Part model, mm, in its own coordinate system. Face numbers are marked on the shaded views. A direction names the side the tool comes from. Coordinates: 2 decimals unless noted, no trailing zeros. Write each loop counter-clockwise with the first axis right and the second up, starting at its lowest first coordinate (ties: lowest second). Pieces come first, ordered by that corner, then holes. Notation, with made-up numbers: (-23, 69) - (25, 69) arc R20 ccw to (25, 98) - close; hole circle Ø6 at (67.25, -17.75). An arc over 180 degrees is marked (long way). Use a Markdown table: item, result.
```python
from build123d import *

# Parameters (mm, degrees)
SKETCH1_R           = 15
SKETCH1_R_2         = 10
BOSS_EXTRUDE1_DEPTH = 5
BOSS_EXTRUDE2_DEPTH = 9.5
FILLET1_R           = 0.5


with BuildPart() as part:
    # Sketch1 → Boss-Extrude1 (new body)
    with BuildSketch(Plane.XY):
        Circle(SKETCH1_R)
        Circle(SKETCH1_R_2, mode=Mode.SUBTRACT)
    extrude(amount=BOSS_EXTRUDE1_DEPTH)

    # Sketch1_3 → Boss-Extrude2 (add)
    with BuildSketch(Plane.XY):
        with BuildLine():
            Line((-9.797958971, 2), (-2, 2))
            Line((-2, 2), (-2, 9.797958971))
            ThreePointArc((-2, 9.797958971), (-7.071067812, 7.071067812), (-9.797958971, 2))
        make_face()
        with BuildLine():
            Line((2, 9.797958971), (2, 2))
            Line((2, 2), (9.797958971, 2))
            ThreePointArc((9.797958971, 2), (7.071067812, 7.071067812), (2, 9.797958971))
        make_face()
        with BuildLine():
            Line((2, -2), (2, -9.797958971))
            ThreePointArc((2, -9.797958971), (7.071067812, -7.071067812), (9.797958971, -2))
            Line((9.797958971, -2), (2, -2))
        make_face()
        with BuildLine():
            ThreePointArc((-9.797958971, -2), (-7.071067812, -7.071067812), (-2, -9.797958971))
            Line((-2, -9.797958971), (-2, -2))
            Line((-2, -2), (-9.797958971, -2))
        make_face()
    extrude(amount=BOSS_EXTRUDE2_DEPTH)

    # Fillet1
    fillet1_edges = [part.edges().sort_by_distance(p)[0] for p in [
        (-2, 5.898979486, 0),
        (-5.898979486, 2, 0),
        (0, 10, 0),
        (5.898979486, 2, 0),
        (2, 5.898979486, 0),
        (10, 0, 0),
        (2, -5.898979486, 0),
        (5.898979486, -2, 0),
        (0, -10, 0),
        (-2, -5.898979486, 0),
        (-5.898979486, -2, 0),
        (-10, 0, 0),
    ]]
    fillet(fillet1_edges, radius=FILLET1_R)


solid = part.part
```
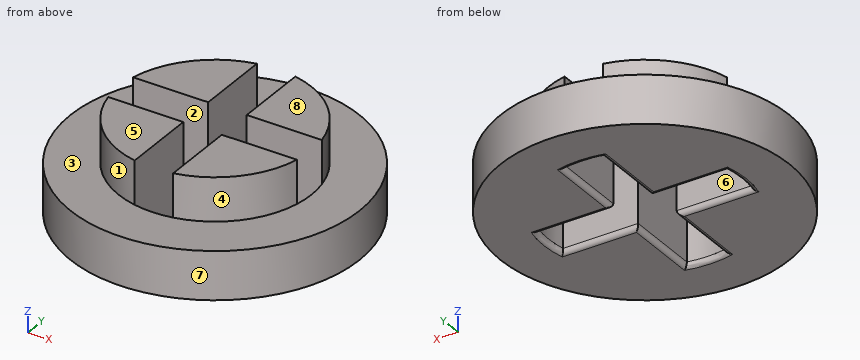
Item 1: Band-saw the part on A-A, the plane z = 3.25. Give the cut face in (x, y).
From the geometry:
| item | result |
|---|---|
| outline | circle Ø30 at (0, 0); hole (-9.8, -2) - (-2, -2) - (-2, -9.8) arc R10 ccw to (2, -9.8) - (2, -2) - (9.8, -2) arc R10 ccw to (9.8, 2) - (2, 2) - (2, 9.8) arc R10 ccw to (-2, 9.8) - (-2, 2) - (-9.8, 2) arc R10 ccw to start |
Item 2: Two-plate mould, pull along X, no slides. Class the marked faces 6, 7 and 8: pulls with the +X half, pulls with the -X half, needs draft (parallel to the pull), parting line crosses it, or undercut.
From the geometry:
| item | result |
|---|---|
| face 6 | undercut |
| face 7 | parting line crosses it |
| face 8 | needs draft |
Item 3: Drop flat-ended pins along their axis: P1, Ø2.5, axis at y = -6.5, z = 5.5, coming from the +X side; P2, Ø1.5, axis at y = 3.5, z = 3.5, coming from the -X side; P3, Ø3, axis at x = -2, z = 6, coming from the -Y side. Give the stop position or say it passes through.
From the geometry:
| item | result |
|---|---|
| P1 | x = 14.01 |
| P2 | x = -14.75 |
| P3 | y = -14.97 |
Item 4: Drill centre lines: probe 1 along Y at (x, z) = (0, 1); probe 2 along Y at (x, z) = (3.5, 7.75); probe 3 along Z at (x, y) = (13, -0.25). Where is each one in solid material? Low to high.
From the geometry:
| item | result |
|---|---|
| probe 1 | -15 to -10, 10 to 15 |
| probe 2 | -9.37 to -2, 2 to 9.37 |
| probe 3 | 0 to 5 |
Item 5: Band-saw the part on C-C, the plane z = 8. Give the cut face in (x, y).
From the geometry:
| item | result |
|---|---|
| outline | (-9.8, -2) arc R10 ccw to (-2, -9.8) - (-2, -2) - close; (-9.8, 2) - (-2, 2) - (-2, 9.8) arc R10 ccw to start; (2, -9.8) arc R10 ccw to (9.8, -2) - (2, -2) - close; (2, 2) - (9.8, 2) arc R10 ccw to (2, 9.8) - close |
Item 6: Which spindle directions (+Z, -Z, +X, -X, +Y, -Y) get a long thin tool onto all of the face, cutting with end or side? Do the marked faces 1, 2, 3, 4 and 5. Say none if no direction does.
From the geometry:
| item | result |
|---|---|
| face 1 | +Z, -X, -Y |
| face 2 | +Z, -Z |
| face 3 | +Z |
| face 4 | +Z, +X, -Y |
| face 5 | +Z, +X, -X, +Y, -Y |
Item 7: Band-saw the part on B-B, the plane y = 0. Give the cut face in (x, z).
From the geometry:
| item | result |
|---|---|
| outline | (-15, 0) - (-10.5, 0) arc R0.5 ccw to (-10, 0.5) - (-10, 5) - (-15, 5) - close; (10, 0.5) arc R0.5 ccw to (10.5, 0) - (15, 0) - (15, 5) - (10, 5) - close |
